Autodesk Inventor part; units mm, degrees
ref_plane "YZ Plane" through (0, 0, 0) normal (1, 0, 0) x (0, 1, 0)
ref_plane "XZ Plane" through (0, 0, 0) normal (0, 1, 0) x (-1, 0, 0)
ref_plane "XY Plane" through (0, 0, 0) normal (0, 0, 1) x (1, 0, 0)
sketch "Sketch1" plane through (0, 0, 0) normal (0, 0, 1) x (1, 0, 0)
  line L0 (0, 0) -> (0, 200)
  line L1 (0, 200) -> (-10, 200)
  line L2 (-10, 200) -> (-200, 10)
  line L3 (-200, 10) -> (-200, 0)
  line L4 (-200, 0) -> (0, 0)
  line L5 (0, 40) -> (-40, 0)
  dimension "d162" = 200
  dimension "d163" = 10
  dimension "d164" = 40
  dimension "d165" = 40
extrude "Plate5" add sketch "Sketch1" along normal blind 4 contours L5 L4 L3 L2 L1 L0
properties part number "PNS-077 stretch plate" material "Stainless Steel"
The listing builds one solid part. Answer for the finished solid, in the listing's coordinates (mm). Round coordinates to 2 decimals unless told otherwise and drop trailing zeros. Order: outer loops, then holes, each group sorted by start corner. A loop starts at its lowest first (then second) coordinate and runs counter-clockwise, first axis right, second up. Notation, with made-up numbers: (84, 86.25) -> (118, 86.25) arc R16 cw to (118, 99.25) -> close; hole circle Ø3 at (38, 83.5). An arc over 180 degrees is marked (long way). Write each question's results on one line, items separated by ' | '. Start each with the question number.
Q1. Find section C-C (x = -144). Determine the outline of the cut face in (y, z).
Q2. Each of these flat-tipped pins is pushed along its axis until it touches: pin 1 (2 mm diameter, centred on y = 157.5, z = 3.5, fed in from -X); pin 2 (1.5 mm diameter, centred on x = -173, z = 1.5, fed in from -Y); pin 3 (1.5 mm diameter, centred on x = -135, z = 0.5, fed in from +Y); pin 4 (2 mm diameter, centred on x = -47.5, z = 2.5, fed in from +Y). Where does it stop, or does it pass through?
Q3. Find section A-A (y = 157). Determine the outline of the cut face in (x, z).
Q4. Find section B-B (z = 2.2). Determine the outline of the cut face in (x, y), then the cut area to 4 significant figures.
Q5. Straight lines are drawn through the part: probe 1 along Y at (x, z) = (-142, 1.65); probe 2 along Y at (x, z) = (-98, 2.2); probe 3 along X at (y, z) = (56.5, 0.45). For each, find the intervals that lie inside material, in ascending order. Write a range as from..to.
Worked answers:
1) outline: (0, 0) -> (66, 0) -> (66, 4) -> (0, 4) -> close
2) pin 1: stops at x = -53.5 | pin 2: stops at y = 0 | pin 3: stops at y = 75.75 | pin 4: stops at y = 163.5
3) outline: (-53, 0) -> (0, 0) -> (0, 4) -> (-53, 4) -> close
4) outline: (-200, 0) -> (-40, 0) -> (0, 40) -> (0, 200) -> (-10, 200) -> (-200, 10) -> close | area: 21,150 mm2
5) probe 1: y = 0..68 | probe 2: y = 0..112 | probe 3: x = -153.5..0
